Geometry: final body of the model. Coordinates: model frame, mm. A direction names the side the tool comes from. Coordinates: 2 decimals unless noted, no trailing zeros. Write each loop counter-clockwise with the first axis right and the second up, starting at its lowest first coordinate (ties: lowest second). Pieces come first, ordered by that corner, then holes. Notation, with made-up numbers: (56.25, 60) - (96.25, 60) arc R30 cw to (96.25, 92) - close; hole circle Ø9 at (21.5, -16.75). An arc over 180 degrees is marked (long way). Answer as a JSON object with one key per item and string values. Group by question number.
Item 1: First-contact query: pin 1 Ø10 at (x, y) = (-143.5, 4087) entering from +Z; pin 2 Ø10 at (x, y) = (-144, 4134) entering from +Z; pin 3 Ø5 at (y, z) = (4146, -100) entering from +X. Flat tips, straight axial feed; report the tip coordinate or a pass-through.
Item 2: Section A-A on x = 0. Return loops of the section in (y, z), and give its area (3 significant figures).
Item 3: Section B-B on z = 0. Return loops of the section in (x, y), and give its area (3 significant figures).
Item 4: Set-up query: faces 4 (the cylindrical face through (-140.858, 3972.627, 108.006)), 5 (the cylindrical face through (-34.685, 4078.88, 156.195)), 6 (the cylindrical face through (137.789, 4181.21, -171.383)). Return all of +Z, -Z, +X, -X, +Y, -Y with unobstructed straight access to the full face (end or side cutting, diameter ignored); none if empty.
Item 5: Section C-C on y = 4102. Return loops of the section in (x, z), and give its area (3 significant figures).
Item 6: Line query: line 1 along X through (y, z) = (4176, 0); line 2 along X through (y, z) = (4173.5, 225); line 3 along Y through (x, z) = (4.5, 2.5). Output: solid intervals per line, ascending. Write a range as from..to.
Item 7: Mould query, pull axis Z, two halves, no side actions, for faces 1 (the cylindrical face through (211.386, 4181.21, 81.243)), 2 (the conical face through (166.24, 4160.29, -52.35)), 3 (the flat face through (77, 4160, 141)). Classes: pulls with the +Z half, pulls with the -Z half, needs draft (parallel to the pull), parting line crosses it, or undercut.
Item 8: Section D-D on y = 3973.5. Return loops of the section in (x, z).
```python
from build123d import *

# Parameters (mm, degrees)
ESBO_O2_R             = 12
CORTE_EXTRUS_O1_DEPTH = 250.990148264


with BuildPart() as part:
    # Esboço1 → Revolução1 (revolve)
    with BuildSketch(Plane.XY):
        with BuildLine():
            Line((0, 4196), (250, 4196))
            Line((250, 4196), (250, 4166))
            Line((250, 4166), (180, 4166))
            Line((180, 4166), (174, 4160))
            Line((174, 4160), (160, 4160))
            Line((160, 4160), (160, 4000))
            Line((160, 4000), (177.5, 4000))
            Line((177.5, 4000), (177.5, 3946.009851736))
            ThreePointArc((177.5, 3946.009851736), (88.77242151, 3949.002336943), (0, 3950))
            Line((0, 3950), (0, 4000))
            Line((0, 4000), (140, 4000))
            Line((140, 4000), (140, 4160))
            Line((140, 4160), (0, 4160))
            Line((0, 4160), (0, 4196))
        make_face()
    revolve(axis=Axis((0, 113.656700564, 0), (0, 1, 0)))

    # Esboço2 → Corte-extrusão1 (cut, through all)
    with BuildSketch(Plane(origin=(0, 4196, 0), x_dir=(1, 0, 0), z_dir=(0, 1, 0))):
        with Locations((0, 225)):
            Circle(ESBO_O2_R)
        with Locations((69.528823734, 213.987716166)):
            Circle(ESBO_O2_R)
        with Locations((132.251681766, 182.028823734)):
            Circle(ESBO_O2_R)
        with Locations((182.028823734, 132.251681766)):
            Circle(ESBO_O2_R)
        with Locations((213.987716166, 69.528823734)):
            Circle(ESBO_O2_R)
        with Locations((225, 0)):
            Circle(ESBO_O2_R)
        with Locations((213.987716166, -69.528823734)):
            Circle(ESBO_O2_R)
        with Locations((182.028823734, -132.251681766)):
            Circle(ESBO_O2_R)
        with Locations((132.251681766, -182.028823734)):
            Circle(ESBO_O2_R)
        with Locations((69.528823734, -213.987716166)):
            Circle(ESBO_O2_R)
        with Locations((0, -225)):
            Circle(ESBO_O2_R)
        with Locations((-69.528823734, -213.987716166)):
            Circle(ESBO_O2_R)
        with Locations((-132.251681766, -182.028823734)):
            Circle(ESBO_O2_R)
        with Locations((-182.028823734, -132.251681766)):
            Circle(ESBO_O2_R)
        with Locations((-213.987716166, -69.528823734)):
            Circle(ESBO_O2_R)
        with Locations((-225, 0)):
            Circle(ESBO_O2_R)
        with Locations((-213.987716166, 69.528823734)):
            Circle(ESBO_O2_R)
        with Locations((-182.028823734, 132.251681766)):
            Circle(ESBO_O2_R)
        with Locations((-132.251681766, 182.028823734)):
            Circle(ESBO_O2_R)
        with Locations((-69.528823734, 213.987716166)):
            Circle(ESBO_O2_R)
    extrude(amount=-CORTE_EXTRUS_O1_DEPTH, mode=Mode.SUBTRACT)


solid = part.part
```
Checks:
{
 "1": {"pin 1": "z = 80.11", "pin 2": "z = 79.24", "pin 3": "x = 126.86"},
 "2": {"outline": "(3946.01, -177.5) - (4000, -177.5) - (4000, -160) - (4160, -160) - (4160, -174) - (4166, -180) - (4166, -213) - (4196, -213) - (4196, 213) - (4166, 213) - (4166, 180) - (4160, 174) - (4160, 160) - (4000, 160) - (4000, 177.5) - (3946.01, 177.5) arc R3950 cw to start; (4166, -250) - (4196, -250) - (4196, -237) - (4166, -237) - close; (4166, 237) - (4196, 237) - (4196, 250) - (4166, 250) - close; hole (4000, -140) - (4160, -140) - (4160, 140) - (4000, 140) - close", "area": "40,300 mm^2"},
 "3": {"outline": "(-250, 4166) - (-237, 4166) - (-237, 4196) - (-250, 4196) - close; (-213, 4166) - (-180, 4166) - (-174, 4160) - (-160, 4160) - (-160, 4000) - (-177.5, 4000) - (-177.5, 3946.01) arc R3950 cw to (177.5, 3946.01) - (177.5, 4000) - (160, 4000) - (160, 4160) - (174, 4160) - (180, 4166) - (213, 4166) - (213, 4196) - (-213, 4196) - close; (237, 4166) - (250, 4166) - (250, 4196) - (237, 4196) - close; hole (-140, 4000) - (140, 4000) - (140, 4160) - (-140, 4160) - close", "area": "40,300 mm^2"},
 "4": {"face 4": "-Y", "face 5": "none", "face 6": "+Y, -Y"},
 "5": {"outline": "circle Ø320 at (0, 0); hole circle Ø280 at (0, 0)", "area": "18,800 mm^2"},
 "6": {"line 1": "-250..-237, -213..213, 237..250", "line 2": "-108.97..-74.3, -64.76..-12, 12..64.76, 74.3..108.97", "line 3": "3950..4000, 4160..4196"},
 "7": {"face 1": "undercut", "face 2": "parting line crosses it", "face 3": "needs draft"},
 "8": {"outline": "circle Ø355 at (0, 0)"}
}
